Input: part model. Units: mm. Frame: model coordinates. A direction names the side the tool comes from. Round coordinates to 2 decimals unless told otherwise and drop trailing zeros. Loops run counter-clockwise (first coordinate to the right, second up) from the corner with the lowest first, then second, coordinate; pieces in that order, holes last. Notation, with made-up numbers: (56.25, 88) -> (95.25, 88) arc R28 cw to (95.25, 108) -> close; hole circle Ø9 at (22, 24.5). An arc over 180 degrees is marked (long way). One line per question, with ' | ' between items. Start each with the question number.
Q1. Mould query, pull axis Y, two halves, no side actions, for faces 1 (the face through (-7, 19, 212.5)), 2 (the face through (-4.336, -19.524, 2.975)). Classes: pulls with the +Y half, pulls with the -Y half, needs draft (parallel to the pull), parting line crosses it, or undercut.
Q2. Cut plane D-D on z = -178. Return loops of the section in (x, y) (3 decimals).
Q3. Cut plane B-B on y = -12. Return loops of the section in (x, z), and give its area (3 significant figures).
Q4. Cut plane C-C on y = 13.5. Return loops of the section in (x, z).
Q5. Access query for faces 3 (the face through (-7, 19, -212.5)), 4 (the face through (-1.7, 20.2, -192.5)). Directions: +Z, -Z, +X, -X, +Y, -Y. A direction counts if a zero-diameter tool reaches every point of the face in a straight line with its end or side. Return the directions, or none.
Q6. Material intervals for L1, parallel to X at y = 0.5, z = 143; L2, parallel to X at y = 1.5, z = 165; L3, parallel to Y at x = -21.2, z = -150, sorted ascending.
Q7. Contact query for flat-ended pins moving along their axis: P1, Ø1.5, axis at y = -18, z = 77, coming from the -X side; P2, Ø3.5, axis at x = 19.5, z = -41, coming from the +Y side; P3, Ø1.5, axis at y = -1.5, z = 105, coming from the -X side; P4, Ø4, axis at y = 10, z = -116.5, coming from the -X side. Output: stop coordinate, or through.
Q8. Cut plane A-A on x = 0. Return loops of the section in (y, z), and give its area (4 significant figures).
Autodesk Inventor part; units mm, degrees
ref_plane "YZ Plane" through (0, 0, 0) normal (1, 0, 0) x (0, 1, 0)
ref_plane "XZ Plane" through (0, 0, 0) normal (0, 1, 0) x (-1, 0, 0)
ref_plane "XY Plane" through (0, 0, 0) normal (0, 0, 1) x (1, 0, 0)
sketch "Sketch1" plane through (0, 0, 0) normal (0, 0, 1) x (1, 0, 0)
  circle A0 centre (0, 0) radius 20
  circle A1 centre (0, 0) radius 23
  dimension "d0" = 40
  dimension "d1" = 46
extrude "Extrusion1" add sketch "Sketch1" along normal mid plane 425
sketch "Sketch2" plane through (0, 0, 0) normal (1, 0, 0) x (0, 1, 0)
  line L0 (0, 280) -> (0, -280)
  line L1 (-280, 0) -> (280, 0)
  point P0 (0, 0)
  point P1 (0, 150)
  point P2 (0, 0)
  point P3 (0, -150)
  dimension "d4" = 150
  dimension "d5" = 150
hole "Hole1" at (0, 0, 150) at (0, 0, 0) at (0, 0, -150) direction (-1, 0, 0) diameter 4.5 end through all
sketch "Sketch3" plane through (0, 0, 0) normal (1, 0, 0) x (0, 1, 0)
  line L0 (23, -192.5) -> (7, -192.5)
  line L1 (7, -192.5) -> (7, 192.5)
  line L2 (7, 192.5) -> (23, 192.5)
  line L3 (23, 192.5) -> (23, -192.5)
  line L4 (23, 212.5) -> (-23, 212.5)
  line L5 (-23, -212.5) -> (23, -212.5)
  line L6 (0, 364) -> (0, -364)
  point P0 (0, 0)
  dimension "d13" = 20
  dimension "d14" = 20
  dimension "d15" = 7
extrude "Extrusion2" cut sketch "Sketch3" along normal through all both and the other way through all
fillet "Fillet1" radius 2 4 edges at (20.3219, 7, -192.5) (-20.3219, 7, -192.5) (20.3219, 7, 192.5) (-20.3219, 7, 192.5)
properties part number "Pancake_Tilt Pipe_4 Lanes" material "PVC-Piping"
Results:
1) face 1: needs draft | face 2: undercut
2) outline: (-21.909, 7) arc R23 ccw (long way) to (21.909, 7) -> (18.735, 7) arc R20 cw (long way) to (-18.735, 7) -> close
3) outline: (-19.62, -212.5) -> (-16, -212.5) -> (-16, 212.5) -> (-19.62, 212.5) -> close; (16, -212.5) -> (19.62, -212.5) -> (19.62, 212.5) -> (16, 212.5) -> close | area: 3,080 mm^2
4) outline: (-18.62, -212.5) -> (-14.76, -212.5) -> (-14.76, -192.5) -> (-18.62, -192.5) -> close; (-18.62, 192.5) -> (-14.76, 192.5) -> (-14.76, 212.5) -> (-18.62, 212.5) -> close; (14.76, -212.5) -> (18.62, -212.5) -> (18.62, -192.5) -> (14.76, -192.5) -> close; (14.76, 192.5) -> (18.62, 192.5) -> (18.62, 212.5) -> (14.76, 212.5) -> close
5) face 3: -Z, +X, -X, +Y, -Y | face 4: +X, -X, +Y
6) L1: -22.99 to -19.99, 19.99 to 22.99 | L2: -22.95 to -19.94, 19.94 to 22.95 | L3: -8.92 to -2.25, 2.25 to 7
7) P1: x = -15.21 | P2: y = 7 | P3: x = -22.99 | P4: through
8) outline: (-23, -212.5) -> (-20, -212.5) -> (-20, 212.5) -> (-23, 212.5) -> close; (20, -212.5) -> (23, -212.5) -> (23, -192.5) -> (20, -192.5) -> close; (20, 192.5) -> (23, 192.5) -> (23, 212.5) -> (20, 212.5) -> close | area: 1,395 mm^2
